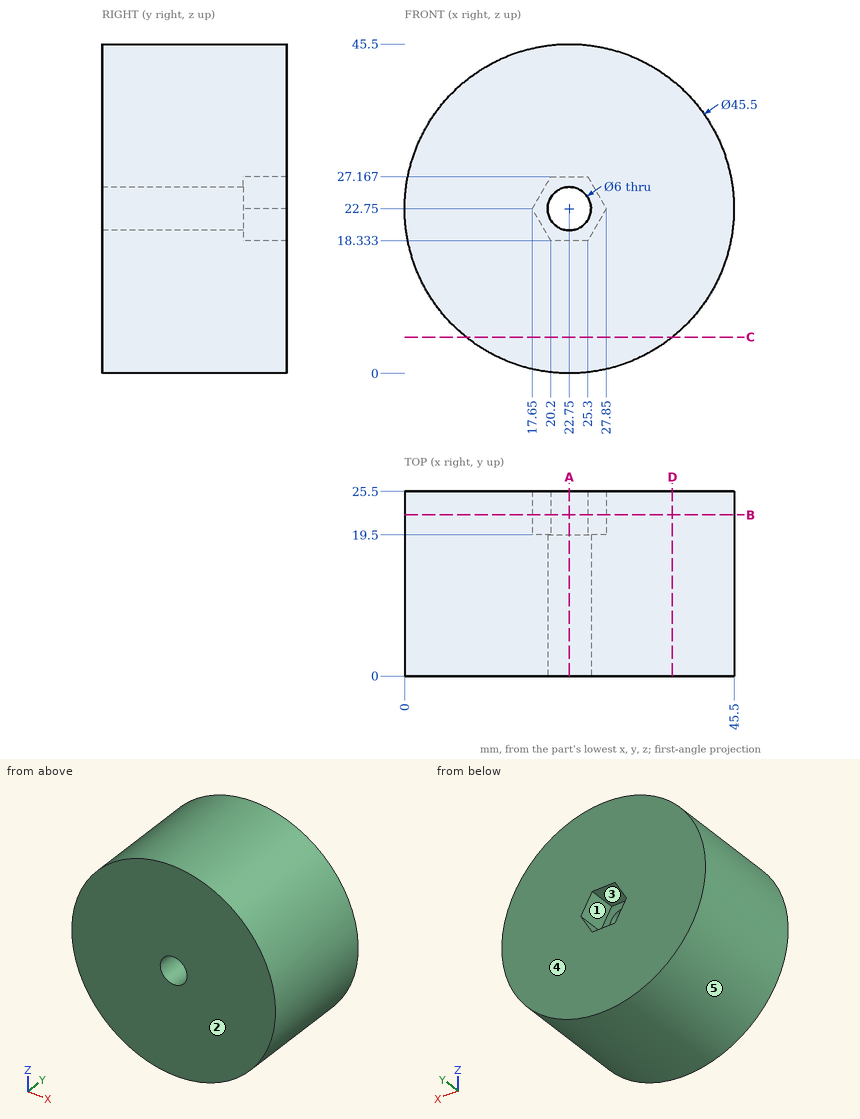
Here's the drawing with two shaded views (mm, measured from the low corner). I have some questions. A direction names the side the tool comes from. Give positions to 0.01 mm unless a question says otherwise; leave off trailing zeros. Order: outer loops, then holes, each group sorted by start corner. A loop starts at its lowest first (then second) coordinate and runs counter-clockwise, first axis right, second up.
Q1. Suppose I cut it at C-C, the plane z = 5. Write out the boundary of the cut face in (x, y).
Q2. For the marked faces 1 and 2, which set-ups out of +Z, -Z, +X, -X, +Y, -Y let a thin tool reach every point of the face, with its end or its side?
Q3. If I drill on line 1 along X through (y, z) = (5.75, 22.75); line 2 along X through (y, z) = (5, 24.5); line 3 along Z through (x, y) = (35.5, 18.75), over which ranges is the centre line in solid material (lowest first)?
Q4. I'm going to push flat-ended pins straight in: P1, Ø3, axis at y = 16, z = 36, coming from the -X side; P2, Ø6, axis at x = 38.5, y = 21, coming from the -Z side; P3, Ø10, axis at y = 8, z = 36.5, coming from the +X side. Where does each tip first touch, or does it pass through?
Q5. We'd pull the mould along Z, two halves only. Please class the marked faces 3, 4 and 5: +Z half, -Z half, draft (parallel to the pull), parting line (faces both ways), or undercut.
Q6. Suppose I cut it at A-A, the plane x = 22.75. Write out the boundary of the cut face in (y, z), and give its area (3 significant figures).
Q7. Suppose I cut it at D-D, the plane x = 37. Write out the boundary of the cut face in (y, z).
Q8. Suppose I cut it at B-B, the plane y = 22.25. Write out the boundary of the cut face in (x, z), and give its area (3 significant figures).
Solution:
1. outline: (8.52, 0) - (36.98, 0) - (36.98, 25.5) - (8.52, 25.5) - close
2. face 1: +Y
2. face 2: +Z, -Z, +X, -X, -Y
3. line 1: x = 0 to 19.75, 25.75 to 45.5
3. line 2: x = 0.07 to 20.31, 25.19 to 45.43
3. line 3: z = 3.91 to 41.59
4. P1: stops at x = 3.27
4. P2: stops at z = 3.91
4. P3: stops at x = 43.75
5. face 3: undercut
5. face 4: draft
5. face 5: parting line
6. outline: (0, 0) - (25.5, 0) - (25.5, 18.33) - (19.5, 18.33) - (19.5, 19.75) - (0, 19.75) - close; (0, 25.75) - (19.5, 25.75) - (19.5, 27.17) - (25.5, 27.17) - (25.5, 45.5) - (0, 45.5) - close
6. area: 990 mm2
7. outline: (0, 5.02) - (25.5, 5.02) - (25.5, 40.48) - (0, 40.48) - close
8. outline: circle Ø45.5 at (22.75, 22.75); hole (17.65, 22.75) - (20.2, 18.33) - (25.3, 18.33) - (27.85, 22.75) - (25.3, 27.17) - (20.2, 27.17) - close
8. area: 1,560 mm2
